```python
from build123d import *

# Parameters (mm, degrees)
F0_W     = 35.1
F0_H     = 2
F1_DEPTH = 95.5
F2_DEPTH = 30
F3_R     = 18
F4_R     = 9.5
F5_R     = 5
F7_D     = 5
F9_D     = 5
F10_R    = 1
F11_R    = 4
F12_R    = 2


with BuildPart() as f1:
    # F0 (on Right) → F1 (new body, symmetric)
    with BuildSketch(Plane.YZ):
        with Locations((36.25, -1)):
            Rectangle(F0_W, F0_H)
    extrude(amount=F1_DEPTH, both=True)

    # F0 (on Right) → F2 (join, symmetric)
    with BuildSketch(Plane.YZ):
        Polygon((18.7, 0), (3.5, 0), (0, 0), (0, -3.5), (0, -90.4), (2, -90.4), (2, -3.5), (2, -2), (3.5, -2), (18.7, -2), align=None)
    extrude(amount=F2_DEPTH, both=True)

    # F3
    f3_edges = [f1.edges().sort_by_distance(p)[0] for p in [
        (95.5, 18.7, -1),
        (-95.5, 18.7, -1),
    ]]
    fillet(f3_edges, radius=F3_R)

    # F4
    f4_edges = [f1.edges().sort_by_distance(p)[0] for p in [
        (-30, 18.7, -1),
        (30, 18.7, -1),
    ]]
    fillet(f4_edges, radius=F4_R)

    # F5
    f5_edges = [f1.edges().sort_by_distance(p)[0] for p in [
        (-30, 1, -90.4),
        (30, 1, -90.4),
    ]]
    fillet(f5_edges, radius=F5_R)

    # F7 (through all)
    with Locations(Plane.XZ):
        with Locations((0, -70.2), (0, -34.9)):
            Hole(F7_D / 2)

    # F9 (through all)
    with Locations(Plane.XY):
        with Locations((-80, 46.6), (0, 46.6), (80, 46.6)):
            Hole(F9_D / 2)

    # F10
    f10_edges = [f1.edges().sort_by_distance(p)[0] for p in [
        (95.5, 53.8, -1),
        (-95.5, 53.8, -1),
    ]]
    fillet(f10_edges, radius=F10_R)

    # F11
    f11_edges = [f1.edges().sort_by_distance(p)[0] for p in [
        (0, 0, 0),
    ]]
    fillet(f11_edges, radius=F11_R)

    # F12
    f12_edges = [f1.edges().sort_by_distance(p)[0] for p in [
        (0, 2, -2),
    ]]
    fillet(f12_edges, radius=F12_R)


solid = f1.part
```
Design review of the part built by this model. Coordinates are the model's own, in mm. A direction names the side the tool comes from. Round coordinates to 2 decimals unless told otherwise and drop trailing zeros. Write each loop counter-clockwise with the first axis right and the second up, starting at its lowest first coordinate (ties: lowest second). Pieces come first, ordered by that corner, then holes.
Item 1: We need section D-D on x = -80. Write out the cut boundary in (y, z), and give its area (3 significant figures).
Item 2: We need section A-A on y = 46.6. Write out the cut boundary in (x, z), and give its area (3 significant figures).
Item 3: For probe 1 along X at (y, z) = (46, -1); probe 2 along X at (y, z) = (1, -70); probe 3 along Y at (x, z) = (8, -27.5), list the stretches that pass through material, from the lowest coordinate up.
Item 4: We need section B-B on z = -34.9. Write out the cut boundary in (x, y), and give its area (3 significant figures).
Item 5: We need section C-C on x = 9. Write out the cut boundary in (y, z), and give its area (3 significant figures).
Item 6: The part is to be moulded in two halves that separate along Y. For faces 4 (the flat face through (0, 2, -48)), 5 (the cylindrical face through (-32.857, 15.991, -0.986)), 6 (the flat face through (-30, 1, -39)), 7 (the cylindrical face through (80.54, 44.16, -1.01)), say which applies: +Y half, -Y half, draft (parallel to the pull), parting line (faces both ways), or undercut.
Item 7: Clearance check with flat-ended pins moving along their axes: pin 1 Ø6 at (x, z) = (0, -70.2) entering from -Y; pin 2 Ø1.6 at (x, z) = (51.5, -1) entering from -Y; pin 3 Ø25 at (x, y) = (23, 31) entering from -Z; pin 4 Ø10 at (y, z) = (5.5, -47.5) entering from +X. State where each tip first meets the part, or that it passes through.
Item 8: For faces 1 (the flat face through (30, 1, -39)), 2 (the flat face through (1, 34, -2)), 3 (the flat face through (1, 34, 0)), list the 3-axis set-ups (+Z, -Z, +X, -X, +Y, -Y) from which the entire face can be reached by the end or side of a thin tool; tool diameter is ignored.
Returned:
1. outline: (18.87, -2) - (44.1, -2) - (44.1, 0) - (18.87, 0) - close; (49.1, -2) - (53.8, -2) - (53.8, 0) - (49.1, 0) - close
1. area: 59.9 mm2
2. outline: (-95.5, -2) - (-82.5, -2) - (-82.5, 0) - (-95.5, 0) - close; (-77.5, -2) - (-2.5, -2) - (-2.5, 0) - (-77.5, 0) - close; (2.5, -2) - (77.5, -2) - (77.5, 0) - (2.5, 0) - close; (82.5, -2) - (95.5, -2) - (95.5, 0) - (82.5, 0) - close
2. area: 352 mm2
3. probe 1: x = -95.5 to -82.43, -77.57 to -2.43, 2.43 to 77.57, 82.43 to 95.5
3. probe 2: x = -30 to -2.49, 2.49 to 30
3. probe 3: y = 0 to 2
4. outline: (-30, 0) - (-2.5, 0) - (-2.5, 2) - (-30, 2) - close; (2.5, 0) - (30, 0) - (30, 2) - (2.5, 2) - close
4. area: 110 mm2
5. outline: (0, -90.4) - (2, -90.4) - (2, -4) arc R2 cw to (4, -2) - (53.8, -2) - (53.8, 0) - (4, 0) arc R4 ccw to (0, -4) - close
5. area: 282 mm2
6. face 4: +Y half
6. face 5: -Y half
6. face 6: draft
6. face 7: undercut
7. pin 1: stops at y = 0
7. pin 2: stops at y = 18.7
7. pin 3: stops at z = -2
7. pin 4: stops at x = 30
8. face 1: +Z, -Z, +X, -Y
8. face 2: -Z, +X, -X, +Y
8. face 3: +Z, +X, -X, +Y, -Y
